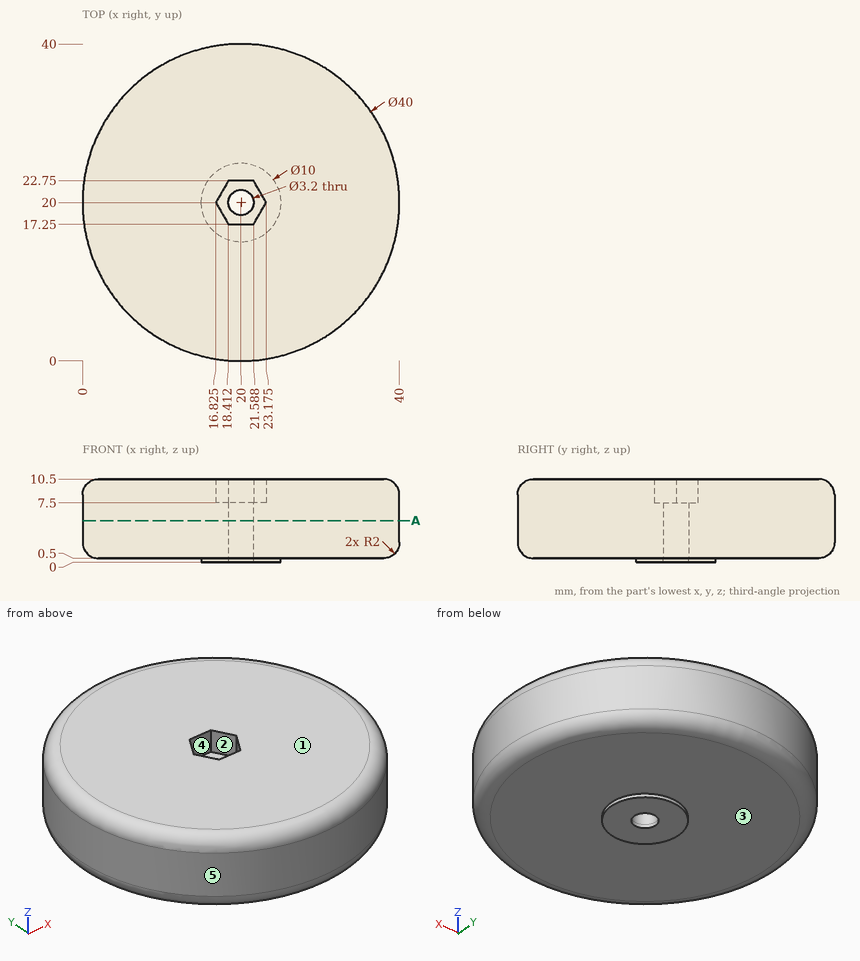
Verification items for this drawing (mm, ordinates from the low corner). A direction names the side the tool comes from. Give positions to 0.01 mm unless a question says otherwise; leave off trailing zeros. Loops run counter-clockwise (first coordinate to the right, second up) from the corner with the lowest first, then second, coordinate; pieces in that order, holes last. Notation, with made-up numbers: M 26,-5 L 72,-5 A18 cw 72,24 Z; hole C 18,46.25 d5. An arc over 180 degrees is marked long. Answer as a JSON object with one key per item and string values. Group by question number.
Item 1: Sectioned sample at A-A on z = 5.25. Record the boundary of the cut face in (x, y), plus the area to 3 significant figures.
Item 2: Material ranges on L1, parallel to Y at x = 20, z = 5; L2, parallel to Y at x = 20, z = 0.2; L3, parallel to Z at x = 21, y = 10, recorded low to high.
Item 3: Access from +Z, -Z, +X, -X, +Y, -Y to the whole of each face (thin tool, end or side, straight path). Record for the marked faces 1 and 2.
Item 4: Mould release check, pull along Y, two halves, no side actions. Record for the marked faces 3, 4 and 5: pulls with the +Y half, pulls with the -Y half, needs draft (parallel to the pull), parting line crosses it, or undercut.
Item 5: Gauge pin test, flat ends, axial feed: pin 1 (1.5 mm diameter, centred on x = 13.5, z = 3.5, fed in from -Y) (1 decimal); pin 2 (1.5 mm diameter, centred on y = 35, z = 8.5, fed in from -X) (1 decimal); pin 3 (3 mm diameter, centred on x = 19.5, z = 7, fed in from -Y); pin 4 (2.5 mm diameter, centred on x = 20, y = 20, fed in from +Z). Record the tip position at first contact, or that the pin passes through.
Findings below:
{
 "1": {"outline": "C 20,20 d40; hole C 20,20 d3.2", "area": "1,250 mm2"},
 "2": {"L1": "0 to 18.4, 21.6 to 40", "L2": "15 to 18.4, 21.6 to 25", "L3": "0.5 to 10.5"},
 "3": {"face 1": "+Z, +X, -X, +Y, -Y", "face 2": "+Z"},
 "4": {"face 3": "needs draft", "face 4": "undercut", "face 5": "parting line crosses it"},
 "5": {"pin 1": "y = 0.8", "pin 2": "x = 6", "pin 3": "y = 0", "pin 4": "through"}
}
